Autodesk Inventor part; units mm, degrees
ref_plane "YZ Plane" through (0, 0, 0) normal (1, 0, 0) x (0, 1, 0)
ref_plane "XZ Plane" through (0, 0, 0) normal (0, 1, 0) x (-1, 0, 0)
ref_plane "XY Plane" through (0, 0, 0) normal (0, 0, 1) x (1, 0, 0)
sketch "Sketch1" plane through (0, 0, 0) normal (0, 1, 0) x (-1, 0, 0)
  circle A0 centre (0, 0) radius 24
  circle A1 centre (0, 0) radius 22
  dimension "d0" = 48
  dimension "d2" = 2
extrude "Extrusion1" add sketch "Sketch1" along normal blind 4
sketch "Sketch2" plane through (0, 4, 0) normal (0, 1, 0) x (1, 0, 0)
  circle A0 centre (0, 0) radius 24
  circle A1 centre (0, 0) radius 22
  circle A2 centre (0, 0) radius 20
  circle A3 centre (0, 0) radius 17
  circle A4 centre (0, 0) radius 14
  circle A5 centre (0, 0) radius 11
  circle A6 centre (0, 0) radius 7
  circle A7 centre (0, 0) radius 4
  dimension "d10" = 40
  dimension "d11" = 48
  dimension "d12" = 44
  dimension "d13" = 34
  dimension "d14" = 28
  dimension "d15" = 22
  dimension "d16" = 14
  dimension "d17" = 8
extrude "Extrusion2" add sketch "Sketch2" against normal blind 1 contours A0 | A1 | A2 | A3 | A4 | A5 | A6 | A7
sketch "Sketch3" plane through (0, 0, 0) normal (0, -1, 0) x (1, 0, 0)
  line L0 (-30, 20) -> (30, 20)
  line L1 (30, 20) -> (30, -20)
  line L2 (30, -20) -> (-30, -20)
  line L3 (-30, -20) -> (-30, 20)
  line L4 (-30, 20) -> (30, -20) construction
  line L5 (30, 20) -> (-30, -20) construction
  point P0 (0, 0)
  dimension "d7" = 60
  dimension "d8" = 40
sketch "Sketch4" plane through (0, 4, 0) normal (0, 1, 0) x (1, 0, 0)
  circle A0 centre (-0.0001, 0.0001) radius 21.6961
  circle A1 centre (-0.0001, 0.0001) radius 19.037
  circle A2 centre (-0.0001, 0.0001) radius 16.6196
  circle A3 centre (-0.0001, 0.0001) radius 11.5431
  circle A4 centre (-0.0001, 0.0001) radius 8.884
  circle A5 centre (-0.0001, 0.0001) radius 13.9605
  line L0 (-0.0001, 21.6962) -> (-0.0001, -21.696) construction
  line L1 (-0.0001, 0.0001) -> (16.9795, -13.5061)
  line L2 (-0.0001, 0.0001) -> (13.057, -17.3272)
  arc A6 (14.8984, -11.8507) -> (16.9795, -13.5061) centre (16.142, -12.4231) ccw
  line L3 (15.9389, -12.6784) -> (16.1106, -12.4626) construction
  arc A7 (10.9255, -8.6905) -> (13.0065, -10.3459) centre (12.1691, -9.2629) ccw
  arc A8 (6.9526, -5.5303) -> (9.0336, -7.1857) centre (8.1962, -6.1027) ccw
  arc A9 (13.057, -17.3272) -> (11.4567, -15.2035) centre (11.9307, -16.5111) ccw
  arc A10 (16.9795, 13.5062) -> (14.8983, 11.8508) centre (16.144, 12.4206) ccw
  line L4 (-0.0001, 0.0001) -> (16.9795, 13.5062)
  arc A11 (13.0065, 10.346) -> (10.9254, 8.6906) centre (12.1712, 9.2602) ccw
  arc A12 (9.0335, 7.1858) -> (6.9525, 5.5304) centre (8.1983, 6.1) ccw
  arc A13 (11.4566, 15.2036) -> (13.057, 17.3274) centre (11.9308, 16.5111) ccw
  line L5 (-0.0001, 0.0001) -> (13.057, 17.3274)
  line L6 (15.9389, 12.6785) -> (16.1126, 12.4601) construction
  line L7 (19.0369, 0.0001) -> (16.6195, 0.0001)
  line L8 (13.9604, 0.0001) -> (11.543, 0.0001)
  line L9 (8.8839, 0.0001) -> (-21.6962, 0.0001)
  line L10 (21.62, -21.5289) -> (21.62, 21.5289)
  line L11 (-0.0001, 0.0001) -> (35.6066, 0.0001)
  line L12 (4.8627, -1.3296) -> (-6.2016, -1.3296)
  line L13 (4.8627, 1.3297) -> (-6.2016, 1.3297)
  line L14 (3.3126, -1.3296) -> (3.3126, 1.3297)
  arc A14 (4.8627, -1.3296) -> (4.8627, 1.3297) centre (4.6178, 0.0001) ccw
  arc A15 (-6.2016, 1.3297) -> (-6.2016, -1.3296) centre (-5.9623, 0.0001) ccw
  point P0 (0, 0)
  point P1 (21.6199, 0.0001)
  point P2 (-0.0001, 21.529)
  point P3 (3.3126, 0.0001)
  point P4 (28.4358, 37.7355)
  point P5 (32.4077, 43.0065)
  point P6 (22.4217, 17.835)
  point P7 (17.2565, 13.7264)
  point P8 (32.2826, 25.6787)
  point P9 (27.1174, 21.5701)
  point P10 (53.6613, 4.5036)
  point P11 (42.1434, 33.5224)
  point P12 (36.9782, 29.4138)
  point P13 (53.6613, -4.5036)
  point P14 (9.0336, 7.1858)
  point P15 (6.9523, 5.5309)
  point P16 (13.0065, 10.346)
  point P17 (10.9252, 8.6911)
  point P18 (11.457, 15.2035)
  point P19 (21.62, -1.8147)
  point P20 (21.62, 1.8149)
  point P21 (14.8981, 11.8513)
  dimension "d18" = 38.074
  dimension "d19" = 2.6591
  dimension "d20" = 2.6591
  dimension "d21" = 2.6591
  dimension "d22" = 2.4174
  dimension "d23" = 2.4174
  dimension "d24" = 1.369
  dimension "d25" = 2.6593
  dimension "d26" = 1.352
  dimension "d27" = 1.351
extrude "Extrusion3" add sketch "Sketch4" along normal blind 2 contours L4 A10 | A0 L10 L11 A1 L4 | L5 A1 L9 A0 | A13 L5 | L9 A1 L2 A0 | L10 A0 L1 A1 L11 | A2 L11 A5 L4 | L4 A11 | L2 A9 | L1 A6 | A2 L1 A5 L11 | A7 L1 | A3 L11 A4 L4 | L4 A12 | A3 L1 A4 L11 | A8 L1 | L13 L14 L9 L4 | L4 L5 L13 | L5 L9 A15 L13 | A14 L12 L14 L9 | L9 L14 L13 A14 | L9 L14 L12 L1 | L1 L12 L2 | L2 L12 A15 L9
extrude "Extrusion4" cut sketch "Sketch3" against normal up to surface (3 mm away)
properties part number "Scanner-Kapak"
The model under review builds one solid part; all positions refer to its coordinate system, in mm. A direction names the side the tool comes from. Round coordinates to 2 decimals unless told otherwise and drop trailing zeros. Write each loop counter-clockwise with the first axis right and the second up, starting at its lowest first coordinate (ties: lowest second). Pieces come first, ordered by that corner, then holes. Notation, with made-up numbers: M 67.5,-13 L 101.5,-13 A26 cw 101.5,6 Z; hole C 63,33.25 d4. An arc over 180 degrees is marked long. Use a Markdown table: item, result. Add a question column.
Q1. We need section B-B, the plane x = 0. State the section outline as (y, z) points.
Q2. Machinability: for faces 4 (the face through (21.62, 5, 0)), 5 (the face through (0, 1, 22)), 6 (the face through (13.96, 4.99, -0.13)), 7 (the face through (11, 1, -20)), which of the approach directions +Z, -Z, +X, -X, +Y, -Y give a long, thin tool a straight path to every point of the face, cutting with its end or side? Answer none if there is none.
Q3. We need section D-D, the plane z = 21. State the section outline as (x, y) points, plus the area to 3 significant figures.
Q4. The part is to be moulded in two halves that separate along X. For faces 1 (the face through (20.13, 4.99, -8.09)), 2 (the face through (-19, 6, -5)), 3 (the face through (-7.313, 4.986, 0.026)), say which applies: pulls with the +X half, pulls with the -X half, needs draft (parallel to the pull), parting line crosses it, or undercut.
Q5. We need section C-C, the plane z = 0. State the section outline as (x, y) points, plus the area to 3 significant figures.
Q6. Insertion check: pin 1 (1.6 mm diameter, centred on y = 5, z = -1, fed in from +X); pin 2 (1 mm diameter, centred on x = 2.5, y = 3, fed in from +Z); pin 3 (1.5 mm diameter, centred on x = -10.5, y = 1.5, fed in from +Z); pin 4 (8 mm diameter, centred on x = 8, z = -3, fed in from +Y). Each pin has a flat end and moves straight along its axis. Give the tip position at first contact, or say it passes through.
Q7. We need section A-A, the plane y = 2.2. State the section outline as (x, z) points.
Q8. To check wall thickness, follow line 1 (X direction, y = 4.85, z = -6.5); line 2 (Z direction, x = 12.5, y = 5.6); line 3 (Z direction, x = 4.5, y = 4.6). State the ranges of each line that lie inside material, in increasing order.
Findings below:
| question | item | result |
|---|---|---|
| 1 | outline | M 0,-24 L 4,-24 L 4,-21.7 L 6,-21.7 L 6,-19.04 L 4,-19.04 L 4,-1.33 L 6,-1.33 L 6,1.33 L 4,1.33 L 4,19.04 L 6,19.04 L 6,21.7 L 4,21.7 L 4,24 L 0,24 L 0,22 L 3,22 L 3,-22 L 0,-22 Z |
| 2 | face 4 | +Z, -Z, +X, +Y |
| 2 | face 5 | -Y |
| 2 | face 6 | +Y |
| 2 | face 7 | +X, -X, -Y |
| 3 | outline | M -11.62,0 L -6.56,0 L -6.56,3 L 6.56,3 L 6.56,0 L 11.62,0 L 11.62,4 L 5.45,4 L 5.45,6 L -5.45,6 L -5.45,4 L -11.62,4 Z |
| 3 | area | 75.4 mm² |
| 4 | face 1 | pulls with the +X half |
| 4 | face 2 | needs draft |
| 4 | face 3 | undercut |
| 5 | outline | M -24,3 L 24,3 L 24,4 L 21.62,4 L 21.62,6 L 19.04,6 L 19.04,4 L 16.62,4 L 16.62,6 L 13.96,6 L 13.96,4 L 11.54,4 L 11.54,6 L 8.88,6 L 8.88,4 L 5.97,4 L 5.97,6 L -7.31,6 L -7.31,4 L -19.04,4 L -19.04,6 L -21.7,6 L -21.7,4 L -24,4 Z |
| 5 | area | 95.7 mm² |
| 6 | pin 1 | stops at x = 21.62 |
| 6 | pin 2 | stops at z = 23.92 |
| 6 | pin 3 | stops at z = 21.93 |
| 6 | pin 4 | stops at y = 6 |
| 7 | outline | M -13.27,-20 A24 ccw 13.27,-20 L 9.17,-20 A22 cw -9.17,-20 Z; M -13.27,20 L -9.17,20 A22 cw 9.17,20 L 13.27,20 A24 ccw Z |
| 8 | line 1 | x = -20.7 to -17.89, 6.89 to 9.54, 12.35 to 15.3, 17.89 to 20.7 |
| 8 | line 2 | z = -17.73 to -15.24, -10.59 to -6.22, 6.22 to 10.59, 15.24 to 17.73 |
| 8 | line 3 | z = -21.22 to -18.5, -1.33 to 1.33, 18.5 to 21.22 |
